from build123d import *

# Parameters (mm, degrees)
CROQUIS1_R              = 1.5
SALIENTE_EXTRUIR1_DEPTH = 10
SALIENTE_EXTRUIR2_START = -5
CROQUIS3_R              = 1.5
SALIENTE_EXTRUIR2_DEPTH = 5
CROQUIS5_W              = 10
CROQUIS5_H              = 12.5
CORTAR_EXTRUIR1_DEPTH   = 16
CROQUIS2_R              = 1.5
SALIENTE_EXTRUIR3_DEPTH = 5
REDONDEO1_R             = 5


with BuildPart() as part:
    # Croquis1 → Saliente-Extruir1 (new body)
    with BuildSketch(Plane.XY):
        with BuildLine():
            Line((5, 0), (5, -125))
            ThreePointArc((5, -125), (0, -130), (-5, -125))
            Line((-5, -125), (-5, 0))
            ThreePointArc((-5, 0), (0, 5), (5, 0))
        make_face()
        Circle(CROQUIS1_R, mode=Mode.SUBTRACT)
        with Locations((0, -125)):
            Circle(CROQUIS1_R, mode=Mode.SUBTRACT)
        with Locations((0, -80)):
            Circle(CROQUIS1_R, mode=Mode.SUBTRACT)
    extrude(amount=SALIENTE_EXTRUIR1_DEPTH)

    # Croquis3 → Saliente-Extruir2 (add)
    with BuildSketch(Plane.XY.offset(SALIENTE_EXTRUIR2_START)):
        with BuildLine():
            Line((-5, -125), (-5, -115))
            Line((-5, -115), (5, -115))
            Line((5, -115), (5, -125))
            ThreePointArc((5, -125), (0, -130), (-5, -125))
        make_face()
        with Locations((0, -125)):
            Circle(CROQUIS3_R, mode=Mode.SUBTRACT)
    extrude(amount=SALIENTE_EXTRUIR2_DEPTH)

    # Croquis5 → Cortar-Extruir1 (cut)
    with BuildSketch(Plane.ZY.offset(5)):
        with Locations((5, -123.75)):
            Rectangle(CROQUIS5_W, CROQUIS5_H)
    extrude(amount=-CORTAR_EXTRUIR1_DEPTH, mode=Mode.SUBTRACT)

    # Croquis2 → Saliente-Extruir3 (add)
    with BuildSketch(Plane.XY.offset(10)):
        with BuildLine():
            Line((-5, -125), (-5, -115))
            Line((-5, -115), (5, -115))
            Line((5, -115), (5, -125))
            ThreePointArc((5, -125), (0, -130), (-5, -125))
        make_face()
        with Locations(Location((0, -125, 0), (0, 0, 180))):
            Circle(CROQUIS2_R, mode=Mode.SUBTRACT)
    extrude(amount=SALIENTE_EXTRUIR3_DEPTH)

    # Redondeo1
    redondeo1_edges = [part.edges().sort_by_distance(p)[0] for p in [
        (0, -115, 10),
        (0, -115, 0),
    ]]
    fillet(redondeo1_edges, radius=REDONDEO1_R - 0.0001)  # a hair under: the kernel refuses the full size


solid = part.part
Input: part model. Units: mm. Frame: model coordinates. A direction names the side the tool comes from. Give positions to 0.01 mm unless a question says otherwise; leave off trailing zeros. Order: outer loops, then holes, each group sorted by start corner. A loop starts at its lowest first (then second) coordinate and runs counter-clockwise, first axis right, second up. Notation, with made-up numbers: M 29,81.5 L 48,81.5 A31 cw 48,119.5 Z; hole C -13.75,29 d6. An arc over 180 degrees is marked long. Answer as a JSON object with one key per item and string values.
1. Cut plane A-A, the plane x = 0. State how many separate pieces and enclosed holes the cut face has, and give its area (3 significant figures).
Result sheet:
{"separate pieces": "5", "enclosed holes": "0", "area": "1,300 mm²"}
2. Reachability of faces 1 (the flat face through (0, -117.5, 5)), 2 (the flat face through (0, -52, 10)), 3 (the cylindrical face through (0, -114, -2)) from +Z, -Z, +X, -X, +Y, -Y: full face, straight path, thin tool, end or side. Return the list, or none.
Result sheet:
{"face 1": "+X, -X, -Y", "face 2": "+Z, +X, -X, +Y", "face 3": "-Z, +X, -X, +Y"}
3. Pull-direction query (X, two-part tool) for faces 4 (the cylindrical face through (0, -130, 12)), 5 (the cylindrical face through (-0.195, -123.513, -2.535)), 6 (the flat face through (0, -52, 0)), 7 (the cylindrical face through (0.806, -78.735, 4.93)); classes: +X half, -X half, draft (parallel to the pull), parting line (faces both ways), or undercut.
Result sheet:
{"face 4": "parting line", "face 5": "undercut", "face 6": "draft", "face 7": "undercut"}
4. Cut plane B-B, the plane y = -80. Output: boundary loops of the cut face in (x, z).
Result sheet:
{"outline": "M -5,0 L -1.5,0 L -1.5,10 L -5,10 Z; M 1.5,0 L 5,0 L 5,10 L 1.5,10 Z"}
5. Ray query, line 1 (Y direction, x = 0, z = 7.25); line 2 (Z direction, x = 1, y = -35); line 3 (X direction, y = -125, z = 12.4). Return the intervals inside material, ascending. Write a range as [from, to].
Result sheet:
{"line 1": "[-117.5, -81.5], [-78.5, -1.5], [1.5, 5]", "line 2": "[0, 10]", "line 3": "[-5, -1.5], [1.5, 5]"}
6. First-contact query: P1, Ø6, axis at x = -3.5, z = 9, coming from the +Y side; P2, Ø1.5, axis at x = 3.5, z = 1.5, coming from the +Y side; P3, Ø1.5, axis at x = -1.5, z = 10.5, coming from the +Y side; P4, Ø2.5, axis at x = 0, y = -80, coming from the -Z side. Flat tips, straight axial feed; report the tip coordinate or a pass-through.
Result sheet:
{"P1": "y = 4.97", "P2": "y = 4.18", "P3": "y = 4.91", "P4": "through"}
7. Cut plane C-C, the plane z = 8. Output: boundary loops of the cut face in (x, y).
Result sheet:
{"outline": "M -5,-117.5 L 5,-117.5 L 5,0 A5 ccw -5,0 Z; hole C 0,-80 d3; hole C 0,0 d3"}
8. Cut plane D-D, the plane y = -64. Output: boundary loops of the cut face in (x, z), and give its area (3 significant figures).
Result sheet:
{"outline": "M -5,0 L 5,0 L 5,10 L -5,10 Z", "area": "100 mm²"}
